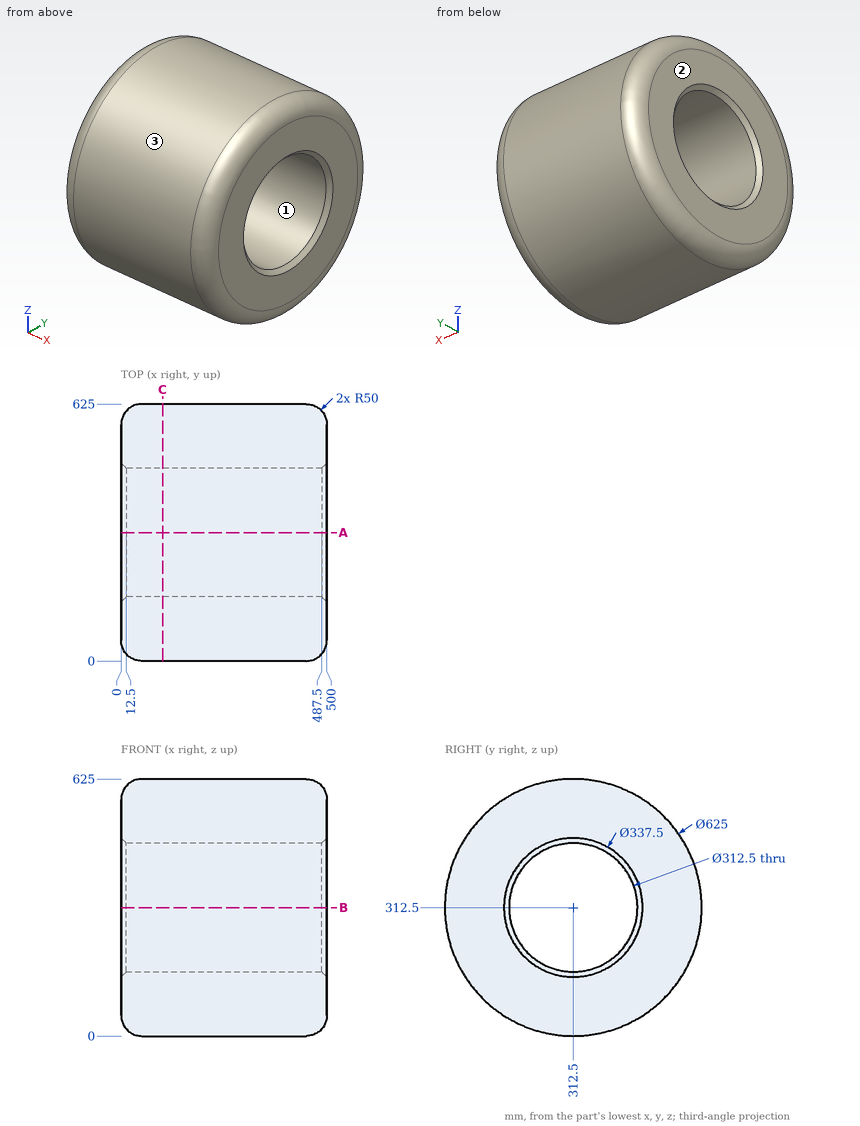
Geometry check sheet. Reference: drawing and pictorial views, mm from the part's lowest x, y, z. Give positions to 0.01 mm unless a question says otherwise; leave off trailing zeros. Order: outer loops, then holes, each group sorted by start corner. A loop starts at its lowest first (then second) coordinate and runs counter-clockwise, first axis right, second up. Notation, with made-up numbers: M 67,46.25 L 99,46.25 A26 cw 99,69.25 Z; hole C 15,4.5 d11. An arc over 180 degrees is marked long. Answer as a JSON object with one key per item and string values. Group by question number.
1) Depth check by flat-ended pin: pin 1 Ø2 at (x, y) = (300.5, 228.5) entering from +Z; pin 2 Ø2 at (x, y) = (421, 135) entering from -Z; pin 3 Ø3 at (x, y) = (108.5, 470.5) entering from +Z. Enter the tip coordinate at first touch or a pass-through.
2) Mould release check, pull along Y, two halves, no side actions. Record for the marked faces 1, 2 and 3: released by +Y, released by -Y, zero draft, split by the parting line, or undercut.
3) Scan lines: line 1 along Y through (x, z) = (297, 312.5); line 2 along Z through (x, y) = (72.5, 359.5). Record each from-to range of solid material in increasing order. Write a range as [from, to].
4) Cross-section at A-A (y = 312.5). Enter the section's corners in (x, z), then the cut area to 3 significant figures.
5) Cross-section at C-C (x = 100.5). Enter the section's corners in (y, z).
Result sheet:
{
 "1": {"pin 1": "stops at z = 613.78", "pin 2": "stops at z = 54.62", "pin 3": "stops at z = 582.99"},
 "2": {"face 1": "undercut", "face 2": "zero draft", "face 3": "split by the parting line"},
 "3": {"line 1": "y = [0, 156.25], [468.75, 625]", "line 2": "z = [3.55, 163.49], [461.51, 621.45]"},
 "4": {"outline": "M 0,50 A50 ccw 50,0 L 450,0 A50 ccw 500,50 L 500,143.75 L 487.5,156.25 L 12.5,156.25 L 0,143.75 Z; M 0,481.25 L 12.5,468.75 L 487.5,468.75 L 500,481.25 L 500,575 A50 ccw 450,625 L 50,625 A50 ccw 0,575 Z", "area": "154,000 mm2"},
 "5": {"outline": "C 312.5,312.5 d625; hole C 312.5,312.5 d312.5"}
}
